Work out the finished part from the listing and answer in its coordinate system (mm). Face numbers are marked on the shaded views. Coordinates: 2 decimals unless noted, no trailing zeros. Order: outer loops, then holes, each group sorted by start corner. A loop starts at its lowest first (then second) coordinate and runs counter-clockwise, first axis right, second up.
1. Determine the mould class of the marked faces 1, 2 and 3 for opening direction Z: +Z half, -Z half, draft (parallel to the pull), parting line (faces both ways), or undercut.
2. The part is cut by section B-B, the plane y = 5.75. Give the vertices of the cut face in (x, z).
3. The part is cut by section D-D, the plane y = 1.5. Give the vertices of the cut face in (x, z), then the cut area to 3 significant figures.
4. The part is cut by section C-C, the plane z = 0. Give the vertices of the cut face in (x, y), then the cut area to 3 significant figures.
5. Flat-ended cylindrical pins translate along their axes: pin 1 Ø0.5 at (y, z) = (6, 22) entering from +X; pin 2 Ø2 at (y, z) = (7, -8.5) entering from -X; pin 3 Ø1.5 at (y, z) = (1, 17) entering from +X. Find the tip coordinate at first contact, or state that the pin passes through.
6. The part is cut by section A-A, the plane x = 0. Give the vertices of the cut face in (y, z).
7. Find the intervals of material crossed by probe 1 along Z at (x, y) = (0, 5.8); probe 2 along Z at (x, y) = (-2, 6.5); probe 3 along Z at (x, y) = (-10.5, 1.5), in increasing order.
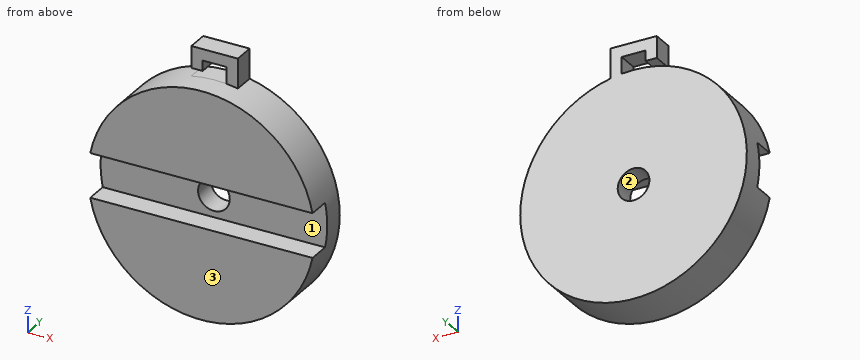
```python
from build123d import *

# Parameters (mm, degrees)
F0_R     = 20
F1_DEPTH = 7.8
F3_DEPTH = 3.9
F4_R     = 2.8
F5_DEPTH = 3.901
F6_W     = 8.2
F6_H     = 5.25
F7_DEPTH = 3.7
F9_DEPTH = 3.701


with BuildPart() as f1:
    # F0 (on Front) → F1 (new body)
    with BuildSketch(Plane.XZ):
        Circle(F0_R)
    extrude(amount=-F1_DEPTH)

    # F2 (on face) → F3 (cut)
    with BuildSketch(Plane.XZ):
        with BuildLine():
            Line((19.6160648449, 3.9), (-19.6160648449, 3.9))
            ThreePointArc((-19.6160648449, 3.9), (-19.903784777, 1.9594263321), (-20, 0))
            ThreePointArc((-20, 0), (-19.903784777, -1.9594263321), (-19.6160648449, -3.9))
            Line((-19.6160648449, -3.9), (19.6160648449, -3.9))
            ThreePointArc((19.6160648449, -3.9), (19.903784777, -1.9594263321), (20, 0))
            ThreePointArc((20, 0), (19.903784777, 1.9594263321), (19.6160648449, 3.9))
        make_face()
    extrude(amount=-F3_DEPTH, mode=Mode.SUBTRACT)

    # F4 (on face) → F5 (cut, through all)
    with BuildSketch(Plane.XZ.offset(-3.9)):
        Circle(F4_R)
    extrude(amount=-F5_DEPTH, mode=Mode.SUBTRACT)

    # F6 (on face) → F7 (join)
    with BuildSketch(Plane(origin=(0, 7.8, 0), x_dir=(-1, 0, 0), z_dir=(0, 1, 0))):
        with Locations((0, 22.2002394621)):
            Rectangle(F6_W, F6_H)
    extrude(amount=-F7_DEPTH)

    # F8 (on face) → F9 (cut, through all)
    with BuildSketch(Plane.XZ.offset(-4.1)):
        with BuildLine():
            Line((-2.1, 22.8252394621), (-2.1, 22.2002394621))
            Line((-2.1, 22.2002394621), (-2.1, 21))
            Line((-2.1, 21), (-4.1, 21))
            Line((-4.1, 21), (-4.1, 19.5752394621))
            ThreePointArc((-4.1, 19.5752394621), (-1.012265376, 19.9743665434), (2.1, 19.8894444367))
            Line((2.1, 19.8894444367), (2.1, 22.8252394621))
            Line((2.1, 22.8252394621), (-2.1, 22.8252394621))
        make_face()
    extrude(amount=-F9_DEPTH, mode=Mode.SUBTRACT)


solid = f1.part
```
Geometry says:
1. face 1: undercut
1. face 2: undercut
1. face 3: draft
2. outline: (-4.1, 21) - (-2.1, 21) - (-2.1, 22.83) - (2.1, 22.83) - (2.1, 19.89) arc R20 ccw (long way) to (4.1, 19.58) - (4.1, 24.83) - (-4.1, 24.83) - close; hole circle Ø5.6 at (0, 0)
3. outline: (-19.62, -3.9) arc R20 ccw to (19.62, -3.9) - close; (-19.62, 3.9) - (19.62, 3.9) arc R20 ccw to start
3. area: 947 mm2
4. outline: (-20, 3.9) - (-2.8, 3.9) - (-2.8, 7.8) - (-20, 7.8) - close; (2.8, 3.9) - (20, 3.9) - (20, 7.8) - (2.8, 7.8) - close
4. area: 134 mm2
5. pin 1: stops at x = 4.1
5. pin 2: stops at x = -18.54
5. pin 3: stops at x = 11.66
6. outline: (0, -20) - (7.8, -20) - (7.8, -2.8) - (3.9, -2.8) - (3.9, -3.9) - (0, -3.9) - close; (0, 3.9) - (3.9, 3.9) - (3.9, 2.8) - (7.8, 2.8) - (7.8, 20) - (0, 20) - close; (4.1, 22.83) - (7.8, 22.83) - (7.8, 24.83) - (4.1, 24.83) - close
7. probe 1: z = -20 to -2.8, 2.8 to 20, 22.83 to 24.83
7. probe 2: z = -19.9 to -1.96, 1.96 to 19.9, 22.83 to 24.83
7. probe 3: z = -17.02 to -3.9, 3.9 to 17.02
